```python
from build123d import *

# Parameters (mm, degrees)
SKETCH_1_W          = 90
SKETCH_1_H          = 71
EXTRUDE_1_DEPTH     = 4
SKETCH_2_R          = 1.5
CUT_EXTRUDE_1_DEPTH = 58.456505289
SKETCH_3_R          = 13
SKETCH_3_R_2        = 1.5
CUT_EXTRUDE_2_DEPTH = 58.456505289


with BuildPart() as part:
    # 草图1 → 凸台-拉伸1 (new body)
    with BuildSketch(Plane.XY):
        Rectangle(SKETCH_1_W, SKETCH_1_H)
    extrude(amount=EXTRUDE_1_DEPTH)

    # 草图2 → 切除-拉伸1 (cut, through all)
    with BuildSketch(Plane.XY.offset(4)):
        with Locations((0, 28)):
            Circle(SKETCH_2_R)
        with Locations((-30, 28)):
            Circle(SKETCH_2_R)
        with Locations(Location((30, 28, 0), (0, 0, 180))):
            Circle(SKETCH_2_R)
    extrude(amount=-CUT_EXTRUDE_1_DEPTH, mode=Mode.SUBTRACT)

    # 草图3 → 切除-拉伸2 (cut, through all)
    with BuildSketch(Plane.XY.offset(4)):
        with Locations((0, -10.5)):
            Circle(SKETCH_3_R)
        with Locations((-31, 4.5)):
            Circle(SKETCH_3_R_2)
        with Locations((-31, -25.5)):
            Circle(SKETCH_3_R_2)
        with Locations((31, -25.5)):
            Circle(SKETCH_3_R_2)
        with Locations((31, 4.5)):
            Circle(SKETCH_3_R_2)
    extrude(amount=-CUT_EXTRUDE_2_DEPTH, mode=Mode.SUBTRACT)


solid = part.part
```
Part model, mm, in its own coordinate system. Give positions to 0.01 mm unless a question says otherwise; leave off trailing zeros. Order: outer loops, then holes, each group sorted by start corner. A loop starts at its lowest first (then second) coordinate and runs counter-clockwise, first axis right, second up. Notation, with made-up numbers: M -23.75,-23.75 L -2.75,-23.75 A19 ccw -2.75,4.25 Z; hole C 18,83 d10. An arc over 180 degrees is marked long. Use a Markdown table: item, result. Add a question column.
(1) Mould opens along X. For faces 1 (the face through (31.11, 26.99, 2.03)), 2 (the face through (-1, 35.5, 2)), 3 (the face through (-45, 0, 2)), 4 (the face through (29.5, 4.57, 2.03)) say: +X half, -X half, draft (parallel to the pull), parting line (faces both ways), or undercut.
(2) Probe line 1 along Y through (x, z) = (0, 0.9); line 2 along Y through (x, z) = (1, 0.55); line 3 along Y through (x, z) = (31, 1.5). List the from-to ranges inside material, lowest first. Write a range as [from, to].
(3) Saw through at B-B, the plane y = 28. Give the cut face in (x, z), and give its area (3 significant figures).
(4) Saw through at A-A, the plane y = 4.5. Give the cut face in (x, z).
(5) Saw through at C-C, the plane z = 2. Give the number of separate pieces and of enclosed holes in the cut face, and give its area (3 significant figures).
(6) Saw through at D-D, the plane y = -10.5. Give the cut face in (x, z), and give its area (3 significant figures).
Answer key:
| question | item | result |
|---|---|---|
| 1 | face 1 | undercut |
| 1 | face 2 | draft |
| 1 | face 3 | -X half |
| 1 | face 4 | undercut |
| 2 | line 1 | [-35.5, -23.5], [2.5, 26.5], [29.5, 35.5] |
| 2 | line 2 | [-35.5, -23.46], [2.46, 26.88], [29.12, 35.5] |
| 2 | line 3 | [-35.5, -27], [-24, 3], [6, 26.88], [29.12, 35.5] |
| 3 | outline | M -45,0 L -31.5,0 L -31.5,4 L -45,4 Z; M -28.5,0 L -1.5,0 L -1.5,4 L -28.5,4 Z; M 1.5,0 L 28.5,0 L 28.5,4 L 1.5,4 Z; M 31.5,0 L 45,0 L 45,4 L 31.5,4 Z |
| 3 | area | 324 mm^2 |
| 4 | outline | M -45,0 L -32.5,0 L -32.5,4 L -45,4 Z; M -29.5,0 L 29.5,0 L 29.5,4 L -29.5,4 Z; M 32.5,0 L 45,0 L 45,4 L 32.5,4 Z |
| 5 | separate pieces | 1 |
| 5 | enclosed holes | 8 |
| 5 | area | 5,810 mm^2 |
| 6 | outline | M -45,0 L -13,0 L -13,4 L -45,4 Z; M 13,0 L 45,0 L 45,4 L 13,4 Z |
| 6 | area | 256 mm^2 |
